Geometry check sheet. Reference: the model listing, model coordinates, mm. Round coordinates to 2 decimals unless told otherwise and drop trailing zeros. Answer as a JSON object with one key per item and string values. Group by question number.
```python
from build123d import *

# Parameters (mm, degrees)
SKETCH_1_W                  = 319
SKETCH_1_H                  = 219
EXTRUDE_1_DEPTH             = 6
HOLE_WIZARD_M41_D           = 3.3
HOLE_WIZARD_M41_CSINK_D     = 4.05
HOLE_WIZARD_M41_CSINK_ANGLE = 90
PATTERN_LINEAR_3_COUNT      = 7
PATTERN_LINEAR_3_PITCH      = 50
PATTERN_LINEAR_3_COUNT_DIR2 = 5
PATTERN_LINEAR_3_PITCH_DIR2 = 50
SKETCH_8_R                  = 2.6
CUT_EXTRUDE_2_DEPTH         = 194.562651356
SKETCH_9_R                  = 2.1
CUT_EXTRUDE_3_DEPTH         = 194.562651356
CHAMFER_1_SIZE              = 2
CHAMFER_1_OF_MIRROR_1_SIZE  = 2


# Read off the part's stored shape, not the designer's step: Зеркальное отражение2
with BuildPart() as part:
    # Эскиз1 → Бобышка-Вытянуть1 (new body)
    with BuildSketch(Plane.XY):
        Rectangle(SKETCH_1_W, SKETCH_1_H)
    extrude(amount=EXTRUDE_1_DEPTH)

    # Отверстие обработанное метчиком M41 (through all)
    with Locations(Plane(origin=(0, 0, 0), x_dir=(-1, 0, 0), z_dir=(0, 0, -1))):
        with Locations((-150, -100)):
            hole_wizard_m41 = CounterSinkHole(HOLE_WIZARD_M41_D / 2, HOLE_WIZARD_M41_CSINK_D / 2, counter_sink_angle=HOLE_WIZARD_M41_CSINK_ANGLE)

    # Линейный массив3: Hole Wizard M41 7 × 5, 8 skipped
    with Locations(*[(-i * PATTERN_LINEAR_3_PITCH, j * PATTERN_LINEAR_3_PITCH_DIR2, 0) for i in range(PATTERN_LINEAR_3_COUNT) for j in range(PATTERN_LINEAR_3_COUNT_DIR2) if (i, j) not in ((0, 0), (1, 1), (1, 3), (2, 2), (3, 1), (3, 3), (4, 2), (5, 1), (5, 3))]):
        add(hole_wizard_m41, mode=Mode.SUBTRACT)

    # Эскиз8 → Вырез-Вытянуть2 (cut, through all)
    with BuildSketch(Plane(origin=(0, 0, 0), x_dir=(-1, 0, 0), z_dir=(0, 0, -1))):
        with Locations((-117, 70)):
            Circle(SKETCH_8_R)
        with Locations((117, 70)):
            Circle(SKETCH_8_R)
        with Locations((117, -70)):
            Circle(SKETCH_8_R)
        with Locations((-117, -70)):
            Circle(SKETCH_8_R)
    extrude(amount=-CUT_EXTRUDE_2_DEPTH, mode=Mode.SUBTRACT)

    # Эскиз9 → Вырез-Вытянуть3 (cut, through all)
    with BuildSketch(Plane(origin=(0, 0, 0), x_dir=(-1, 0, 0), z_dir=(0, 0, -1))):
        with Locations((-127.359161028, 79.417419116)):
            Circle(SKETCH_9_R)
        with Locations((-103.664695294, 74.262587054)):
            Circle(SKETCH_9_R)
        with Locations((-119.976143679, 56.31999383)):
            Circle(SKETCH_9_R)
    cut_extrude_3 = extrude(amount=-CUT_EXTRUDE_3_DEPTH, mode=Mode.SUBTRACT)

    # Фаска1
    chamfer_1_edges = [part.edges().sort_by_distance(p)[0] for p in [
        (129.459161028, 79.417419116, 6),
        (105.764695294, 74.262587054, 6),
        (122.076143679, 56.31999383, 6),
    ]]
    chamfer(chamfer_1_edges, length=CHAMFER_1_SIZE)

    # Зеркальное отражение1: Вырез-Вытянуть3 across plane
    add(cut_extrude_3.mirror(Plane(origin=(0, 0, 0), x_dir=(0, 0, 1), z_dir=(1, 0, 0))), mode=Mode.SUBTRACT)

    # Фаска1 of Зеркальное отражение1
    chamfer_1_of_mirror_1_edges = [part.edges().sort_by_distance(p)[0] for p in [
        (-129.459161028, 79.417419116, 6),
        (-105.764695294, 74.262587054, 6),
        (-122.076143679, 56.31999383, 6),
    ]]
    chamfer(chamfer_1_of_mirror_1_edges, length=CHAMFER_1_OF_MIRROR_1_SIZE)

    # Зеркальное отражение2 outline → Зеркальное отражение2 (revolve, cut)
    with BuildSketch(Plane(origin=(127.359161028, -79.417419116, 0), x_dir=(1, 0, 0), z_dir=(0, -1, 0))):
        Polygon((4.1, 6), (0, 6), (0, 0), (2.1, 0), (2.1, 4), align=None)
    revolve(axis=Axis((127.359161028, -79.417419116, 0), (0, 0, 1)), mode=Mode.SUBTRACT)

    # Mirror 2 2 outline → Mirror 2 2 (revolve, cut)
    with BuildSketch(Plane(origin=(103.664695294, -74.262587054, 0), x_dir=(1, 0, 0), z_dir=(0, -1, 0))):
        Polygon((4.1, 6), (0, 6), (0, 0), (2.1, 0), (2.1, 4), align=None)
    revolve(axis=Axis((103.664695294, -74.262587054, 0), (0, 0, 1)), mode=Mode.SUBTRACT)

    # Mirror 2 3 outline → Mirror 2 3 (revolve, cut)
    with BuildSketch(Plane(origin=(119.976143679, -56.31999383, 0), x_dir=(1, 0, 0), z_dir=(0, -1, 0))):
        Polygon((4.1, 6), (0, 6), (0, 0), (2.1, 0), (2.1, 4), align=None)
    revolve(axis=Axis((119.976143679, -56.31999383, 0), (0, 0, 1)), mode=Mode.SUBTRACT)

    # Mirror 2 4 outline → Mirror 2 4 (revolve, cut)
    with BuildSketch(Plane(origin=(-127.359161028, -79.417419116, 0), x_dir=(1, 0, 0), z_dir=(0, -1, 0))):
        Polygon((4.1, 6), (0, 6), (0, 0), (2.1, 0), (2.1, 4), align=None)
    revolve(axis=Axis((-127.359161028, -79.417419116, 0), (0, 0, 1)), mode=Mode.SUBTRACT)

    # Mirror 2 5 outline → Mirror 2 5 (revolve, cut)
    with BuildSketch(Plane(origin=(-103.664695294, -74.262587054, 0), x_dir=(1, 0, 0), z_dir=(0, -1, 0))):
        Polygon((4.1, 6), (0, 6), (0, 0), (2.1, 0), (2.1, 4), align=None)
    revolve(axis=Axis((-103.664695294, -74.262587054, 0), (0, 0, 1)), mode=Mode.SUBTRACT)

    # Mirror 2 6 outline → Mirror 2 6 (revolve, cut)
    with BuildSketch(Plane(origin=(-119.976143679, -56.31999383, 0), x_dir=(1, 0, 0), z_dir=(0, -1, 0))):
        Polygon((4.1, 6), (0, 6), (0, 0), (2.1, 0), (2.1, 4), align=None)
    revolve(axis=Axis((-119.976143679, -56.31999383, 0), (0, 0, 1)), mode=Mode.SUBTRACT)


solid = part.part
```
1) Thickness scan on line 1 along X through (y, z) = (-50, 2.4); line 2 along Y through (x, z) = (-50, 3.6); line 3 along X through (y, z) = (0, 2.8). Record the ranges inside material, lowest first. Write a range as [from, to].
2) Release check for a two-part mould opening along X. For faces 1 (the flat face through (-2, 2, 6)), 2 (the conical face through (102.02, -72.76, 4.13)), 3 (the conical face through (-121.742, -57.674, 4.125)), 4 (the flat face through (-159.5, -2, 3)) record: +X half, -X half, draft (parallel to the pull), parting line (faces both ways), or undercut.
3) Go/stop test with flat-tipped pins: P1, Ø4, axis at x = -100, y = 0, coming from the -Z side (3 decimals); P2, Ø2.5, axis at x = 50, y = 50, coming from the +Z side. Record where each tip stops, or that it passes through.
Final values:
{
 "1": {"line 1": "x = [-159.5, -151.65], [-148.35, -51.65], [-48.35, 48.35], [51.65, 148.35], [151.65, 159.5]", "line 2": "y = [-109.5, -101.65], [-98.35, -51.65], [-48.35, 48.35], [51.65, 98.35], [101.65, 109.5]", "line 3": "x = [-159.5, -151.65], [-148.35, -101.65], [-98.35, -1.65], [1.65, 98.35], [101.65, 148.35], [151.65, 159.5]"},
 "2": {"face 1": "draft", "face 2": "undercut", "face 3": "undercut", "face 4": "-X half"},
 "3": {"P1": "stops at z = 0.025", "P2": "passes through"}
}
